Print and shaded views of the part. All mm, measured from the part's lowest x, y and z. A direction names the side the tool comes from. Coordinates: 2 decimals unless noted, no trailing zeros. Loops run counter-clockwise (first coordinate to the right, second up) from the corner with the lowest first, then second, coordinate; pieces in that order, holes last. Notation, with made-up numbers: M 69,71 L 116,71 A19 ccw 116,95 Z; hole C 20.25,1 d7. An arc over 180 degrees is marked long. Answer as a JSON object with one key per item and string values. Group by question number.
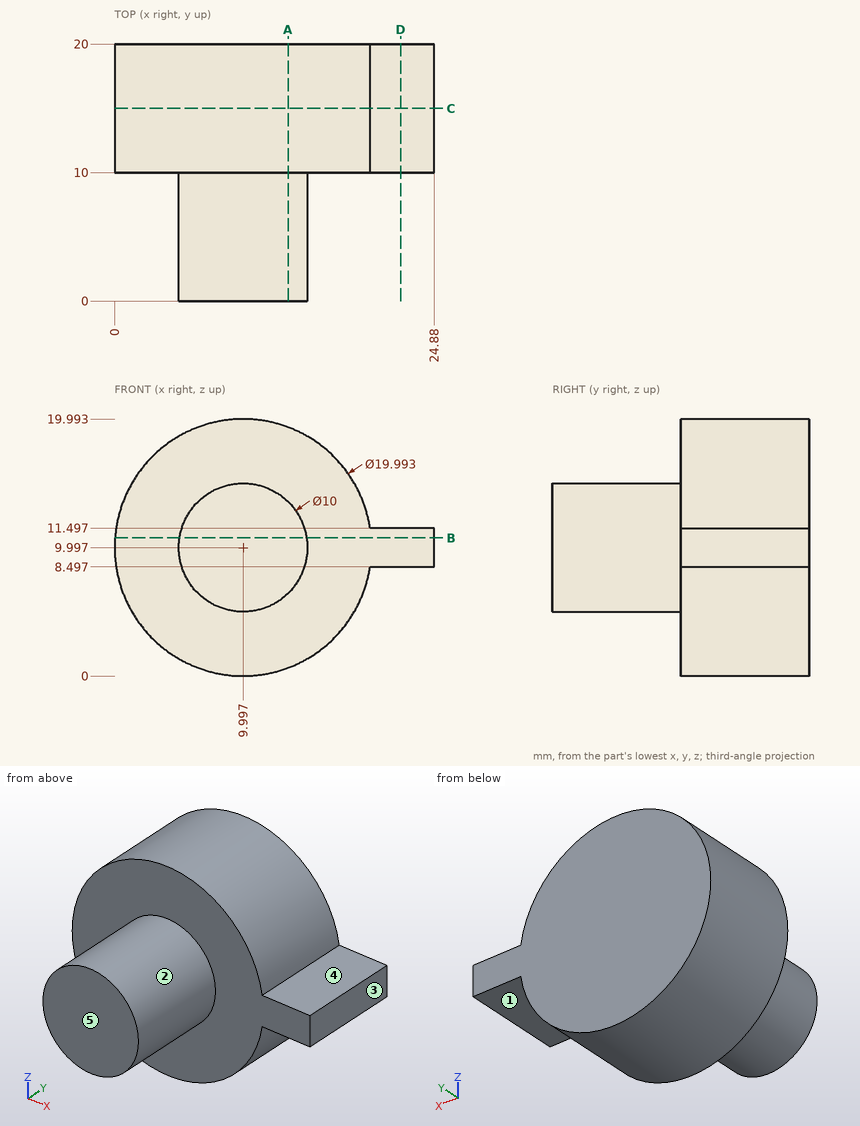
Item 1: Pin check, flat tips, straight feed: pin 1 (5.5 mm diameter, centred on x = 22, y = 12.5, fed in from -Z) (1 decimal); pin 2 (1 mm diameter, centred on x = 3.5, y = 8, fed in from -Z); pin 3 (6 mm diameter, centred on x = 3.5, z = 2.5, fed in from -Y); pin 4 (8 mm diameter, centred on y = 8, z = 17, fed in from +X) (1 decimal). Stop position of each tip, or through.
Item 2: Drill centre lines: L1, parallel to Y at x = 6.75, z = 1.5; L2, parallel to X at y = 3.25, z = 10; L3, parallel to Z at x = 21.25, y = 17. Where is each one in solid material? Low to high. Write a range as from..to.
Item 3: Tool access for the marked faces 1, 2, 3, 4 and 5: list every direction of +Z, -Z, +X, -X, +Y, -Y with a clear straight run to the whole face (end or side of a thin tool).
Item 4: Slice it at B-B, the plane z = 10.75. Write the cut outline in (x, y), then the cut area to 3 significant figures.
Item 5: Slice it at A-A, the plane x = 13.5. Write the cut outline in (y, z) (1 decimal), then the cut area to 3 significant figures.
Item 6: Slice it at C-C, the plane y = 15. Write the cut outline in (x, z).
Item 7: Slice it at D-D, the plane x = 22.25. Write the cut outline in (y, z).
Computed:
{
 "1": {"pin 1": "z = 6.2", "pin 2": "through", "pin 3": "y = 10", "pin 4": "x = 19.3"},
 "2": {"L1": "10..20", "L2": "5..15", "L3": "8.5..11.5"},
 "3": {"face 1": "-Z, +X, +Y, -Y", "face 2": "-Y", "face 3": "+Z, -Z, +X, +Y, -Y", "face 4": "+Z, +X, +Y, -Y", "face 5": "+Z, -Z, +X, -X, -Y"},
 "4": {"outline": "M 0.03,10 L 5.05,10 L 5.05,0 L 14.94,0 L 14.94,10 L 24.88,10 L 24.88,20 L 0.03,20 Z", "area": "347 mm2"},
 "5": {"outline": "M 0,6.4 L 10,6.4 L 10,0.6 L 20,0.6 L 20,19.4 L 10,19.4 L 10,13.6 L 0,13.6 Z", "area": "259 mm2"},
 "6": {"outline": "M 19.88,8.5 L 24.88,8.5 L 24.88,11.5 L 19.88,11.5 A10 ccw long Z"},
 "7": {"outline": "M 10,8.5 L 20,8.5 L 20,11.5 L 10,11.5 Z"}
}
